Autodesk Inventor part; units mm, degrees
ref_plane "YZ Plane" through (0, 0, 0) normal (1, 0, 0) x (0, 1, 0)
ref_plane "XZ Plane" through (0, 0, 0) normal (0, 1, 0) x (-1, 0, 0)
ref_plane "XY Plane" through (0, 0, 0) normal (0, 0, 1) x (1, 0, 0)
sketch "Sketch1" plane through (0, 0, 0) normal (0, 0, 1) x (1, 0, 0)
  arc A0 (10.377, 42.8791) -> (11.579, 42.394) centre (10.6, 41.7) ccw
  arc A1 (10.1355, 44.1565) -> (12.9139, 42.6464) centre (10.6, 41.7) ccw
  arc A2 (20.2623, 33.4501) -> (21.2356, 30.5256) centre (18.8812, 31.3663) ccw
  line L0 (10.1355, 44.1565) -> (14.0658, 44.8997)
  line L1 (14.0658, 44.8997) -> (23.9257, 38.0598)
  line L2 (23.9257, 38.0598) -> (21.2356, 30.5256)
  line L3 (10.377, 42.8791) -> (13.7723, 43.5211)
  line L4 (13.7723, 43.5211) -> (22.4517, 37.5001)
  line L5 (22.4517, 37.5001) -> (20.1055, 30.9291)
  line L6 (11.579, 42.394) -> (12.9139, 42.6464)
  line L7 (20.2623, 33.4501) -> (19.834, 32.2506)
  arc A3 (19.834, 32.2506) -> (20.1055, 30.9291) centre (18.8812, 31.3663) ccw
  line L8 (10.6, 41.7) -> (18.8812, 31.3663) construction
  point P0 (0, 0)
  dimension "d0" = 5
  dimension "d1" = 5
  dimension "d2" = 1.3
  dimension "d5" = 1.3
  dimension "d6" = 12
  dimension "d7" = 4
  dimension "d8" = 8
  dimension "d9" = 0.7
  dimension "d10" = 0.7
  dimension "d11" = 62
  dimension "d12" = 1.2
extrude "Extrusion1" add sketch "Sketch1" along normal mid plane 10
fillet "Fillet1" radius 2 2 edges at (22.4517, 37.5001, 0) (13.7723, 43.5211, 0)
fillet "Fillet1" radius 3 2 edges at (14.0658, 44.8997, 0) (23.9257, 38.0598, 0)
properties part number "Linkage for inset hinge" material "Steel"
Design review of the part built by this model. Coordinates are the model's own, in mm. A direction names the side the tool comes from. Round coordinates to 2 decimals unless told otherwise and drop trailing zeros. Write each loop counter-clockwise with the first axis right and the second up, starting at its lowest first coordinate (ties: lowest second). Pieces come first, ordered by that corner, then holes.
Item 1: Wall thickness on L1, parallel to Y at x = 19, z = 2.75; L2, parallel to Y at x = 19.5, z = 4; L3, parallel to X at y = 41.75, z = 1.25: over which ranges is each line inside the solid? List them lowest first.
Item 2: Consider section A-A on x = 18. Give the boundary of the cut face in (y, z).
Item 3: Draft analysis for pull direction Y (two halves, no side actions). For faces 3 (the flat face through (20, 40, -5)), 4 (the flat face through (12.24, 42.52, -0.07)), 5 (the cylindrical face through (13.997, 44.656, -0.07)), state which applies: released by +Y, released by -Y, zero draft, split by the parting line, or undercut.
Item 4: For faces 1 (the flat face through (20.05, 32.86, -0.07)), 2 (the flat face through (20, 40, 5)), list the 3-axis set-ups (+Z, -Z, +X, -X, +Y, -Y) from which the entire face can be reached by the end or side of a thin tool; tool diameter is ignored.
Item 5: For pin 1 Ø3 at (x, y) = (16, 40) entering from -Z; pin 2 Ø1.5 at (y, z) = (38, -1.5) entering from +X; pin 3 Ø2 at (x, z) = (21, -0.5) entering from -Y; pin 4 Ø1.5 at (y, z) = (32.5, -0.5) entering from +X, all flat-tipped, find the tip position at first contact; note any pin that passes through.
Item 6: Consider section D-D on x = 21.5. Give the boundary of the cut face in (y, z), and give its area (3 significant figures).
Item 7: Consider section C-C on z = 2.5. Give the boundary of the cut face in (x, y).
Item 8: Consider section B-B on y = 39.75. Give the boundary of the cut face in (x, z).
Check values:
1. L1: y = 28.87 to 30.07, 32.66 to 33.86, 39.89 to 41.48
1. L2: y = 28.94 to 30.22, 32.51 to 33.79, 39.55 to 41.13
1. L3: x = 8.1 to 9.4, 11.8 to 13.1, 16.33 to 18.61
2. outline: (29.03, -5) - (30.41, -5) - (30.41, 5) - (29.03, 5) - close; (32.32, -5) - (33.71, -5) - (33.71, 5) - (32.32, 5) - close; (40.59, -5) - (42.17, -5) - (42.17, 5) - (40.59, 5) - close
3. face 3: zero draft
3. face 4: undercut
3. face 5: released by +Y
4. face 1: +Z, -Z
4. face 2: +Z, +X, -X, +Y, -Y
5. pin 1: passes through
5. pin 2: stops at x = 23.31
5. pin 3: stops at y = 29.13
5. pin 4: stops at x = 22.21
6. outline: (31.27, -5) - (34.83, -5) - (34.83, 5) - (31.27, 5) - close; (38.11, -5) - (39.74, -5) - (39.74, 5) - (38.11, 5) - close
6. area: 52.0 mm2
7. outline: (10.14, 44.16) arc R2.5 ccw (long way) to (12.91, 42.65) - (11.58, 42.39) arc R1.2 cw (long way) to (10.38, 42.88) - (12.95, 43.37) arc R2 cw to (14.46, 43.04) - (21.19, 38.37) arc R2 cw to (21.94, 36.06) - (20.11, 30.93) arc R1.3 cw (long way) to (19.83, 32.25) - (20.26, 33.45) arc R2.5 ccw (long way) to (21.24, 30.53) - (23.15, 35.9) arc R3 ccw to (22.04, 39.37) - (15.1, 44.18) arc R3 ccw to (12.83, 44.67) - close
8. outline: (9.04, -5) - (12.16, -5) - (12.16, 5) - (9.04, 5) - close; (19.21, -5) - (21.49, -5) - (21.49, 5) - (19.21, 5) - close
